```python
from build123d import *

# Parameters (mm, degrees)
BOSS_EXTRUDE1_DEPTH             = 4.826
M3X0_5_TAPPED_HOLE1_D           = 2.5
TAP_DRILL_FOR_M3X0_5_TAP1_D     = 2.5
TAP_DRILL_FOR_M3X0_5_TAP1_DEPTH = 5
TAP_DRILL_FOR_M3X0_5_TAP1_TIP   = 0.751075774
M3X0_5_TAPPED_HOLE2_D           = 2.5
SKETCH1_3_R                     = 2
BOSS_EXTRUDE2_DEPTH             = 4.826
FILLET1_R                       = 1
M1_TAPPED_HOLES_D               = 1.6
FILLET2_R                       = 1


with BuildPart() as part:
    # Sketch1 → Boss-Extrude1 (new body)
    with BuildSketch(Plane.XY):
        Polygon((-11, 0), (0, 0), (11, 0), (11, 6), (0, 15), (0, 15.837292271), (-5.5, 15.837292271), (-5.5, 15), (-11, 15), align=None)
    extrude(amount=BOSS_EXTRUDE1_DEPTH)

    # M3x0.5 Tapped Hole1 (through all)
    with Locations(Plane.XY.offset(4.826)):
        with Locations((-5.5, 10)):
            Hole(M3X0_5_TAPPED_HOLE1_D / 2)

    # Tap Drill for M3x0.5 Tap1
    with Locations(Plane(origin=(-4, 0, 2.413), x_dir=(0, 0, -1), z_dir=(0, -1, 0))):
        with Locations((0, 0), (0, 12)):
            Hole(TAP_DRILL_FOR_M3X0_5_TAP1_D / 2, depth=TAP_DRILL_FOR_M3X0_5_TAP1_DEPTH)
            with Locations((0, 0, -(TAP_DRILL_FOR_M3X0_5_TAP1_DEPTH + TAP_DRILL_FOR_M3X0_5_TAP1_TIP / 2))):  # 118° drill point
                Cone(0, TAP_DRILL_FOR_M3X0_5_TAP1_D / 2, TAP_DRILL_FOR_M3X0_5_TAP1_TIP, mode=Mode.SUBTRACT)

    # M3x0.5 Tapped Hole2 (through all)
    with Locations(Plane(origin=(-2.6, 12.97, 0), x_dir=(-1, 0, 0), z_dir=(0, 0, -1))):
        with Locations((0, 0)):
            Hole(M3X0_5_TAPPED_HOLE2_D / 2)

    # Sketch1<3> → Boss-Extrude2 (add)
    with BuildSketch(Plane.XY):
        Polygon((-19, 0), (-11, 0), (-11, 15), (-19, 15), (-31, 15), (-31, -3.3), (-19, -3.3), align=None)
        with Locations((-26.2, 9.2)):
            Circle(SKETCH1_3_R, mode=Mode.SUBTRACT)
    extrude(amount=BOSS_EXTRUDE2_DEPTH)

    # Fillet1
    # the kernel refuses this fillet: 1 mm, written as the material it adds along each edge
    with BuildSketch(Plane(origin=(-5.5, 15, 0), x_dir=(-1, 0, 0), z_dir=(0, 0, 1))) as fillet1_piece_1:
        with BuildLine():
            CenterArc((0.98667431, -1), FILLET1_R, 90, 80.635902393)
            Line((0, -0.837292271), (0, 0))
            Line((0, 0), (0.98667431, 0))
        make_face()
    extrude(amount=4.826)
    with BuildSketch(Plane(origin=(0, 15, 0), x_dir=(0, 1, 0), z_dir=(0, 0, 1))) as fillet1_piece_2:
        with BuildLine():
            CenterArc((FILLET1_R * 0.473879127596, -FILLET1_R), FILLET1_R, 90, 50.710593137)
            Line((-FILLET1_R * 0.300078171608, -FILLET1_R * 0.366762209743), (0, 0))
            Line((0, 0), (FILLET1_R * 0.473879127596, 0))
        make_face()
    extrude(amount=4.826)
    # the kernel refuses this fillet: 1 mm, written as the material it takes off along each edge
    with BuildSketch(Plane(origin=(-31, 15, -2.5), x_dir=(1, 0, 0), z_dir=(0, 0, 1)), Plane(origin=(-19, -3.3, -2.5), x_dir=(-1, 0, 0), z_dir=(0, 0, 1)), Plane(origin=(-31, -3.3, -2.5), x_dir=(0, 1, 0), z_dir=(0, 0, 1))) as fillet1_2_piece_1:
        with BuildLine():
            CenterArc((FILLET1_R, -FILLET1_R), FILLET1_R, 90, 90)
            Line((0, -FILLET1_R), (0, 0))
            Line((0, 0), (FILLET1_R, 0))
        make_face()
    extrude(amount=9.826, mode=Mode.SUBTRACT)
    with BuildSketch(Plane(origin=(11, 6, -1.184697819), x_dir=(0, -1, 0), z_dir=(0, 0, 1))) as fillet1_2_piece_2:
        with BuildLine():
            CenterArc((FILLET1_R * 0.473879127596, -FILLET1_R), FILLET1_R, 90, 50.710593137)
            Line((-FILLET1_R * 0.300078171608, -FILLET1_R * 0.366762209743), (0, 0))
            Line((0, 0), (FILLET1_R * 0.473879127596, 0))
        make_face()
    extrude(amount=7.195395638, mode=Mode.SUBTRACT)

    # M1 Tapped Holes (through all)
    with Locations(Plane.XY.offset(4.826)):
        with Locations((-20.9, 12.5), (-20.9, 7)):
            Hole(M1_TAPPED_HOLES_D / 2)

    # Fillet2
    fillet2_edges = [part.edges().sort_by_distance(p)[0] for p in [
        (0, 15.837292271, 2.413),
        (-5.5, 15.837292271, 2.413),
    ]]
    fillet(fillet2_edges, radius=FILLET2_R)


solid = part.part
```
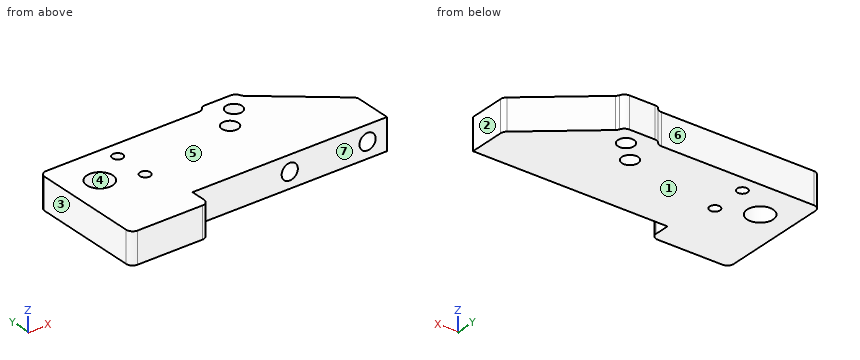
Check sheet for the modelled part. Datum: model origin and axes. Units: mm. Face numbers are marked on the shaded views. A direction names the side the tool comes from. Round coordinates to 2 decimals unless told otherwise and drop trailing zeros. Order: outer loops, then holes, each group sorted by start corner. A loop starts at its lowest first (then second) coordinate and runs counter-clockwise, first axis right, second up. Notation, with made-up numbers: M 27.5,23.5 L 85.5,23.5 A17 cw 85.5,44.5 Z; hole C 42.5,39 d6. An arc over 180 degrees is marked long. Answer in a Markdown table with one row per item.
(1) Section check C-C on z = 4.15. Give the number of separate pieces and of enclosed holes in the cut face, plus the area to 3 significant figures.
Findings:
| item | result |
|---|---|
| separate pieces | 1 |
| enclosed holes | 5 |
| area | 598 mm^2 |
(2) Gauge pin test, flat ends, axial feed: pin 1 (1.5 mm diameter, centred on x = 6.5, z = 3.5, fed in from +Y); pin 2 (2.5 mm diameter, centred on y = -1.5, z = 2.5, fed in from +X); pin 3 (2.5 mm diameter, centred on x = -20, z = 3, fed in from +Y); pin 4 (2 mm diameter, centred on x = -5.5, y = 10, fed in from +Z). Record the tip position at first contact, or that the pin passes through.
Findings:
| item | result |
|---|---|
| pin 1 | stops at y = 10.3 |
| pin 2 | stops at x = -19 |
| pin 3 | stops at y = 15 |
| pin 4 | passes through |
(3) Section check B-B on y = 9.2. Record the boundary of the cut face in (x, z).
Findings:
| item | result |
|---|---|
| outline | M -31,0 L -28.2,0 L -28.2,4.83 L -31,4.83 Z; M -24.2,0 L -6.46,0 L -6.46,4.83 L -24.2,4.83 Z; M -4.54,0 L 7.09,0 L 7.09,4.83 L -4.54,4.83 Z |
(4) Material ranges on line 1 along Y through (x, z) = (-20.9, 1.25); line 2 along X through (y, z) = (3.5, 2.85); line 3 along X through (y, z) = (0.5, 3.05), recorded low to high. Write a range as from..to.
Findings:
| item | result |
|---|---|
| line 1 | y = -3.3..6.2, 7.8..11.7, 13.3..15 |
| line 2 | x = -31..-5.17, -2.83..6.83, 9.17..11 |
| line 3 | x = -31..-5.08, -2.92..6.92, 9.08..11 |
(5) Section check A-A on x = -25. Record the boundary of the cut face in (y, z).
Findings:
| item | result |
|---|---|
| outline | M -3.3,0 L 7.6,0 L 7.6,4.83 L -3.3,4.83 Z; M 10.8,0 L 15,0 L 15,4.83 L 10.8,4.83 Z |
(6) Section check D-D on y = -1.75. Record the boundary of the cut face in (x, z).
Findings:
| item | result |
|---|---|
| outline | M -31,0 L -19,0 L -19,4.83 L -31,4.83 Z |
(7) Set-up check for the marked faces 5, 6 and 7: record each of +Z, -Z, +X, -X, +Y, -Y from which the full face is reachable in a straight line by a thin tool's end or side.
Findings:
| item | result |
|---|---|
| face 5 | +Z, +X, -X, +Y, -Y |
| face 6 | +Z, -Z, -X, +Y |
| face 7 | +Z, -Z, +X, -Y |
(8) Draft check along X on the marked faces 1, 2, 3 and 4. Enter one of: +X half, -X half, draft (parallel to the pull), parting line (faces both ways), or undercut.
Findings:
| item | result |
|---|---|
| face 1 | draft |
| face 2 | +X half |
| face 3 | -X half |
| face 4 | undercut |
